Solid Edge part; units mm, degrees
sketch "Sketch1" plane through (0, 0, 0) normal (0, 0, 1) x (1, 0, 0)
  circle A0 centre (0, 0) radius 60
extrude "Protrusion1" add sketch "Sketch1" against normal blind 25
sketch "Sketch2" plane through (0, 0, 0) normal (0, 0, 1) x (1, 0, 0)
  line L0 (-31.8, -31.8) -> (31.8, -31.8)
  line L1 (31.8, -31.8) -> (31.8, 31.8)
  line L2 (31.8, 31.8) -> (-31.8, 31.8)
  line L3 (-31.8, 31.8) -> (-31.8, -31.8)
extrude "ExtrudedCutout_1" cut sketch "Sketch2" against normal blind 25
sketch "Sketch3" plane through (0, 0, 0) normal (0, 0, 1) x (0, 1, 0)
  circle A0 centre (31.8, 31.8) radius 2.5
  circle A1 centre (-31.8, 31.8) radius 2.5
  circle A2 centre (31.8, -31.8) radius 2.5
  circle A3 centre (-31.8, -31.8) radius 2.5
extrude "ExtrudedCutout_2" cut sketch "Sketch3" against normal blind 25
Build history of the part. All positions in model axes, mm. A direction names the side the tool comes from. Round coordinates to 2 decimals unless told otherwise and drop trailing zeros. Loops run counter-clockwise (first coordinate to the right, second up) from the corner with the lowest first, then second, coordinate; pieces in that order, holes last. Notation, with made-up numbers: (22.5, 59) -> (65.5, 59) arc R24 ccw to (65.5, 94) -> close; hole circle Ø10 at (24, -23). An arc over 180 degrees is marked (long way). One line per item, written item: value. Start each with the question number.
Q1. Probe line 1 along Y through (x, z) = (18, -17.25); line 2 along Y through (x, z) = (-12.5, -12.25); line 3 along X through (y, z) = (13, -14). List the from-to ranges inside material, lowest first.
Q2. 3-axis set-ups, long thin cutter, end or side, ignore diameter. For faces 1 (the face through (0, -31.8, -12)), 2 (the face through (-1, -39, 0)): which of +Z, -Z, +X, -X, +Y, -Y reach the whole face in a straight line?
Q3. Cut at A-A on z = -12.5. List the corners of the cut face in (x, y).
Q4. Cut at B-B on x = 0. List the corners of the cut face in (y, z), plus the area to 3 significant figures.
Q5. Two-plate mould, pull along X, no slides. Class faces 3 (the face through (33.509, -33.625, -12.325)), 4 (the face through (-1, -39, -25)), 5 (the face through (-59.94, 2.64, -12.32)): released by +X, released by -X, zero draft, split by the parting line, or undercut.
Q6. Drop flat-ended pins along their axis: pin 1 Ø6 at (x, y) = (31.8, -31.8) entering from -Z; pin 2 Ø7.5 at (y, z) = (14.5, -13.5) entering from +X; pin 3 Ø12 at (x, z) = (-25, -9) entering from -Y; pin 4 Ø3 at (y, z) = (-33.5, -21) entering from +X. Give the stop position or say it passes through.
Q7. Cut at D-D on x = 47.5. List the corners of the cut face in (y, z), plus the area to 3 significant figures.
Q8. Cut at C-C on y = -10.5. List the corners of the cut face in (x, z).
Computed:
1. line 1: -57.24 to -31.8, 31.8 to 57.24
1. line 2: -58.68 to -31.8, 31.8 to 58.68
1. line 3: -58.57 to -31.8, 31.8 to 58.57
2. face 1: +Z, -Z
2. face 2: +Z, +X, -X, +Y, -Y
3. outline: circle Ø120 at (0, 0); hole (-31.8, -29.3) arc R2.5 ccw (long way) to (-29.3, -31.8) -> (29.3, -31.8) arc R2.5 ccw (long way) to (31.8, -29.3) -> (31.8, 29.3) arc R2.5 ccw (long way) to (29.3, 31.8) -> (-29.3, 31.8) arc R2.5 ccw (long way) to (-31.8, 29.3) -> close
4. outline: (-60, -25) -> (-31.8, -25) -> (-31.8, 0) -> (-60, 0) -> close; (31.8, -25) -> (60, -25) -> (60, 0) -> (31.8, 0) -> close
4. area: 1,410 mm²
5. face 3: undercut
5. face 4: zero draft
5. face 5: split by the parting line
6. pin 1: z = -25
6. pin 2: x = 59.03
6. pin 3: y = -56.91
6. pin 4: x = 50.75
7. outline: (-36.66, -25) -> (36.66, -25) -> (36.66, 0) -> (-36.66, 0) -> close
7. area: 1,830 mm²
8. outline: (-59.07, -25) -> (-31.8, -25) -> (-31.8, 0) -> (-59.07, 0) -> close; (31.8, -25) -> (59.07, -25) -> (59.07, 0) -> (31.8, 0) -> close
